The listing builds one solid part. Answer for the finished solid, in the listing's coordinates (mm). Face numbers are marked on the shaded views. Give positions to 0.01 mm unless a question says otherwise; leave off trailing zeros. Answer in a Markdown table with one row per item.
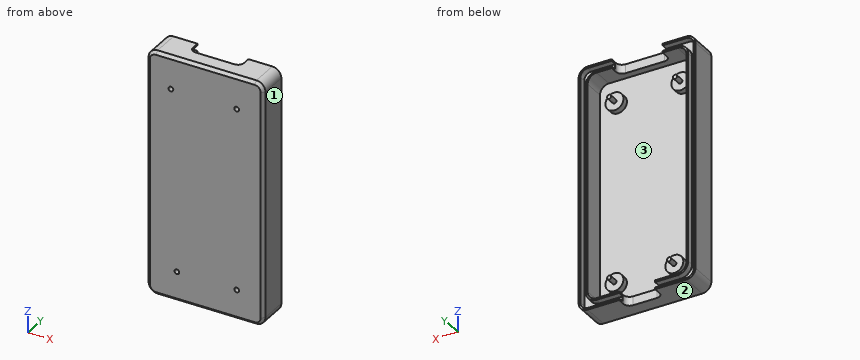
from build123d import *

# Parameters (mm, degrees)
SKETCH1_W                       = 39
SKETCH1_H                       = 81.75
SKETCH1_R                       = 3
BOSS_EXTRUDE1_DEPTH             = 3
SKETCH3_W                       = 39
SKETCH3_H                       = 81.75
SKETCH3_W_2                     = 33
SKETCH3_H_2                     = 75.75
BOSS_EXTRUDE3_DEPTH             = 5
BOSS_EXTRUDE4_START             = 3
SKETCH1_3_R                     = 3
BOSS_EXTRUDE4_DEPTH             = 2
SKETCH8_R                       = 0.7
BOARD_MOUNTING_STANDOFFS_DEPTH  = 3
TAP_DRILL_FOR_M2X0_4_TAP1_D     = 1.6
TAP_DRILL_FOR_M2X0_4_TAP1_DEPTH = 4.519311505
TAP_DRILL_FOR_M2X0_4_TAP1_TIP   = 0.480688495
FILLET2_R                       = 3
SKETCH6_W                       = 12
SKETCH6_H                       = 3
SKETCH6_W_2                     = 17
CUT_EXTRUDE1_DEPTH              = 2.5
STANDOFFS1_LIP_START            = 8
STANDOFFS1_LIP_DEPTH            = 2
STANDOFFS2_LIP_START            = 8
STANDOFFS2_LIP_DEPTH            = 2
FILLET4_R                       = 2
CHAMFER1_SIZE                   = 1


with BuildPart() as part:
    # Sketch1 → Boss-Extrude1 (new body)
    # profile 1 of 5: a face of its own
    with BuildSketch(Plane(origin=(0, 0, 0), x_dir=(1, 0, 0), z_dir=(0, 1, 0))):
        with Locations((14.5, 35.875)):
            Rectangle(SKETCH1_W, SKETCH1_H)
        with Locations((3, 6)):
            Circle(SKETCH1_R, mode=Mode.SUBTRACT)
        with Locations((25, 6)):
            Circle(SKETCH1_R, mode=Mode.SUBTRACT)
        with Locations((5, 66.75)):
            Circle(SKETCH1_R, mode=Mode.SUBTRACT)
        with Locations((25, 66.75)):
            Circle(SKETCH1_R, mode=Mode.SUBTRACT)
    # profile 2 of 5: a face of its own
    with BuildSketch(Plane(origin=(0, 0, 0), x_dir=(1, 0, 0), z_dir=(0, 1, 0))):
        with Locations((5, 66.75)):
            Circle(SKETCH1_R)
    # profile 3 of 5: a face of its own
    with BuildSketch(Plane(origin=(0, 0, 0), x_dir=(1, 0, 0), z_dir=(0, 1, 0))):
        with Locations((25, 66.75)):
            Circle(SKETCH1_R)
    # profile 4 of 5: a face of its own
    with BuildSketch(Plane(origin=(0, 0, 0), x_dir=(1, 0, 0), z_dir=(0, 1, 0))):
        with Locations((25, 6)):
            Circle(SKETCH1_R)
    # profile 5 of 5: a face of its own
    with BuildSketch(Plane(origin=(0, 0, 0), x_dir=(1, 0, 0), z_dir=(0, 1, 0))):
        with Locations((3, 6)):
            Circle(SKETCH1_R)
    extrude(amount=BOSS_EXTRUDE1_DEPTH)

    # Sketch3 → Boss-Extrude3 (add)
    with BuildSketch(Plane(origin=(0, 3, 0), x_dir=(1, 0, 0), z_dir=(0, 1, 0))):
        with Locations((14.5, 35.875)):
            Rectangle(SKETCH3_W, SKETCH3_H)
        with Locations((14.5, 35.875)):
            Rectangle(SKETCH3_W_2, SKETCH3_H_2, mode=Mode.SUBTRACT)
    extrude(amount=BOSS_EXTRUDE3_DEPTH)

    # Sketch1<3> → Boss-Extrude4 (add)
    with BuildSketch(Plane(origin=(0, 0, 0), x_dir=(1, 0, 0), z_dir=(0, 1, 0)).offset(BOSS_EXTRUDE4_START)):
        with Locations(Location((3, 6, 0), (0, 0, 270))):
            Circle(SKETCH1_3_R)
        with Locations(Location((25, 6, 0), (0, 0, 270))):
            Circle(SKETCH1_3_R)
        with Locations(Location((25, 66.75, 0), (0, 0, 270))):
            Circle(SKETCH1_3_R)
        with Locations(Location((5, 66.75, 0), (0, 0, 270))):
            Circle(SKETCH1_3_R)
    extrude(amount=BOSS_EXTRUDE4_DEPTH)

    # Sketch8 → Board Mounting Standoffs (add)
    with BuildSketch(Plane(origin=(0, 5, 0), x_dir=(1, 0, 0), z_dir=(0, 1, 0))):
        with Locations(Location((5, 66.75, 0), (0, 0, 270))):
            Circle(SKETCH8_R)
        with Locations(Location((25, 66.75, 0), (0, 0, 270))):
            Circle(SKETCH8_R)
        with Locations(Location((3, 6, 0), (0, 0, 270))):
            Circle(SKETCH8_R)
        with Locations(Location((25, 6, 0), (0, 0, 270))):
            Circle(SKETCH8_R)
    extrude(amount=BOARD_MOUNTING_STANDOFFS_DEPTH)

    # Tap Drill for M2x0.4 Tap1
    with Locations(Plane(origin=(0, 0, 0), x_dir=(-1, 0, 0), z_dir=(0, -1, 0))):
        with Locations((-25, 66.75), (-5, 66.75), (-25, 6), (-3, 6)):
            Hole(TAP_DRILL_FOR_M2X0_4_TAP1_D / 2, depth=TAP_DRILL_FOR_M2X0_4_TAP1_DEPTH)
            with Locations((0, 0, -(TAP_DRILL_FOR_M2X0_4_TAP1_DEPTH + TAP_DRILL_FOR_M2X0_4_TAP1_TIP / 2))):  # 118° drill point
                Cone(0, TAP_DRILL_FOR_M2X0_4_TAP1_D / 2, TAP_DRILL_FOR_M2X0_4_TAP1_TIP, mode=Mode.SUBTRACT)

    # Fillet2
    fillet2_edges = [part.edges().sort_by_distance(p)[0] for p in [
        (-2, 5.5, -73.75),
        (-2, 5.5, 2),
        (31, 5.5, 2),
        (31, 5.5, -73.75),
        (-5, 4, -76.75),
        (34, 4, -76.75),
        (34, 4, 5),
        (-5, 4, 5),
    ]]
    fillet(fillet2_edges, radius=FILLET2_R)

    # Sketch6 → Cut-Extrude1 (cut)
    with BuildSketch(Plane(origin=(0, 8, 0), x_dir=(1, 0, 0), z_dir=(0, 1, 0))):
        with Locations((14.5, 75.25)):
            Rectangle(SKETCH6_W, SKETCH6_H)
        with Locations((14.5, -3.5)):
            Rectangle(SKETCH6_W_2, SKETCH6_H)
    extrude(amount=-CUT_EXTRUDE1_DEPTH, mode=Mode.SUBTRACT)

    # Standoffs1-Lip: read off the stored shape, not the designer's step
    # Standoffs1-Lip outline → Standoffs1-Lip (add)
    with BuildSketch(Plane(origin=(0, 0, 0), x_dir=(1, 0, 0), z_dir=(0, 1, 0)).offset(STANDOFFS1_LIP_START)):
        with BuildLine():
            Line((23, -5), (31, -5))
            ThreePointArc((31, -5), (33.121320344, -4.121320344), (34, -2))
            Line((34, -2), (34, 73.75))
            ThreePointArc((34, 73.75), (33.121320344, 75.871320344), (31, 76.75))
            Line((31, 76.75), (20.5, 76.75))
            Line((20.5, 76.75), (20.5, 73.75))
            Line((20.5, 73.75), (28, 73.75))
            ThreePointArc((28, 73.75), (30.121320344, 72.871320344), (31, 70.75))
            Line((31, 70.75), (31, 1))
            ThreePointArc((31, 1), (30.121320344, -1.121320344), (28, -2))
            Line((28, -2), (23, -2))
            Line((23, -2), (23, -5))
        make_face()
    extrude(amount=STANDOFFS1_LIP_DEPTH)

    # Standoffs1-Lip 2: loft between two sections, ruled curve by curve
    standoffs1_lip_2_from = [
        Edge.make_three_point_arc((33.3, 8, -73.75), (32.626345597, 8, -75.376345597), (31, 8, -76.05)),
        Edge.make_three_point_arc((31, 8, 4.3), (32.626345597, 8, 3.626345597), (33.3, 8, 2)),
        Edge.make_three_point_arc((31.7, 8, -1), (30.61629509, 8, 1.61629509), (28, 8, 2.7)),
        Edge.make_three_point_arc((28, 8, -74.45), (30.61629509, 8, -73.36629509), (31.7, 8, -70.75)),
        Edge.make_line((20.5, 8, -76.05), (31, 8, -76.05)),
        Edge.make_line((33.3, 8, -73.75), (33.3, 8, 2)),
        Edge.make_line((31, 8, 4.3), (23, 8, 4.3)),
        Edge.make_line((20.5, 8, -74.45), (28, 8, -74.45)),
        Edge.make_line((28, 8, 2.7), (23, 8, 2.7)),
        Edge.make_line((31.7, 8, -70.75), (31.7, 8, -1)),
        Edge.make_line((20.5, 8, -74.45), (20.5, 8, -76.05)),
        Edge.make_line((23, 8, 2.7), (23, 8, 4.3)),
    ]
    standoffs1_lip_2_to = [
        Edge.make_three_point_arc((33.404815559, 10, -73.75), (32.700461389, 10, -75.450461389), (31, 10, -76.154815559)),
        Edge.make_three_point_arc((31, 10, 4.404815559), (32.700461389, 10, 3.700461389), (33.404815559, 10, 2)),
        Edge.make_three_point_arc((31.595184441, 10, -1), (30.542179298, 10, 1.542179298), (28, 10, 2.595184441)),
        Edge.make_three_point_arc((28, 10, -74.345184441), (30.542179298, 10, -73.292179298), (31.595184441, 10, -70.75)),
        Edge.make_line((20.5, 10, -76.154815559), (31, 10, -76.154815559)),
        Edge.make_line((33.404815559, 10, -73.75), (33.404815559, 10, 2)),
        Edge.make_line((31, 10, 4.404815559), (23, 10, 4.404815559)),
        Edge.make_line((20.5, 10, -74.345184441), (28, 10, -74.345184441)),
        Edge.make_line((28, 10, 2.595184441), (23, 10, 2.595184441)),
        Edge.make_line((31.595184441, 10, -70.75), (31.595184441, 10, -1)),
        Edge.make_line((20.5, 10, -74.345184441), (20.5, 10, -76.154815559)),
        Edge.make_line((23, 10, 2.595184441), (23, 10, 4.404815559)),
    ]
    standoffs1_lip_2 = Solid(Shell([*[Face.make_surface_from_curves(standoffs1_lip_2_from[k], standoffs1_lip_2_to[k]) for k in range(12)], Face(Wire(standoffs1_lip_2_from)), Face(Wire(standoffs1_lip_2_to))]))
    add(standoffs1_lip_2, mode=Mode.SUBTRACT)

    # Standoffs2-Lip: read off the stored shape, not the designer's step
    # Standoffs2-Lip outline → Standoffs2-Lip (add)
    with BuildSketch(Plane(origin=(0, 0, 0), x_dir=(1, 0, 0), z_dir=(0, 1, 0)).offset(STANDOFFS2_LIP_START)):
        with BuildLine():
            ThreePointArc((-2, 76.75), (-4.121320344, 75.871320344), (-5, 73.75))
            Line((-5, 73.75), (-5, -2))
            ThreePointArc((-5, -2), (-4.121320344, -4.121320344), (-2, -5))
            Line((-2, -5), (6, -5))
            Line((6, -5), (6, -2))
            Line((6, -2), (1, -2))
            ThreePointArc((1, -2), (-1.121320344, -1.121320344), (-2, 1))
            Line((-2, 1), (-2, 70.75))
            ThreePointArc((-2, 70.75), (-1.121320344, 72.871320344), (1, 73.75))
            Line((1, 73.75), (8.5, 73.75))
            Line((8.5, 73.75), (8.5, 76.75))
            Line((8.5, 76.75), (-2, 76.75))
        make_face()
    extrude(amount=STANDOFFS2_LIP_DEPTH)

    # Standoffs2-Lip 2: loft between two sections, ruled curve by curve
    standoffs2_lip_2_from = [
        Edge.make_three_point_arc((-4.3, 8, 2), (-3.626345597, 8, 3.626345597), (-2, 8, 4.3)),
        Edge.make_three_point_arc((-2, 8, -76.05), (-3.626345597, 8, -75.376345597), (-4.3, 8, -73.75)),
        Edge.make_three_point_arc((-2.7, 8, -70.75), (-1.61629509, 8, -73.36629509), (1, 8, -74.45)),
        Edge.make_three_point_arc((1, 8, 2.7), (-1.61629509, 8, 1.61629509), (-2.7, 8, -1)),
        Edge.make_line((-2, 8, -76.05), (8.5, 8, -76.05)),
        Edge.make_line((6, 8, 4.3), (-2, 8, 4.3)),
        Edge.make_line((1, 8, -74.45), (8.5, 8, -74.45)),
        Edge.make_line((6, 8, 2.7), (1, 8, 2.7)),
        Edge.make_line((-4.3, 8, 2), (-4.3, 8, -73.75)),
        Edge.make_line((-2.7, 8, -1), (-2.7, 8, -70.75)),
        Edge.make_line((8.5, 8, -74.45), (8.5, 8, -76.05)),
        Edge.make_line((6, 8, 2.7), (6, 8, 4.3)),
    ]
    standoffs2_lip_2_to = [
        Edge.make_three_point_arc((-4.404815559, 10, 2), (-3.700461389, 10, 3.700461389), (-2, 10, 4.404815559)),
        Edge.make_three_point_arc((-2, 10, -76.154815559), (-3.700461389, 10, -75.450461389), (-4.404815559, 10, -73.75)),
        Edge.make_three_point_arc((-2.595184441, 10, -70.75), (-1.542179298, 10, -73.292179298), (1, 10, -74.345184441)),
        Edge.make_three_point_arc((1, 10, 2.595184441), (-1.542179298, 10, 1.542179298), (-2.595184441, 10, -1)),
        Edge.make_line((-2, 10, -76.154815559), (8.5, 10, -76.154815559)),
        Edge.make_line((6, 10, 4.404815559), (-2, 10, 4.404815559)),
        Edge.make_line((1, 10, -74.345184441), (8.5, 10, -74.345184441)),
        Edge.make_line((6, 10, 2.595184441), (1, 10, 2.595184441)),
        Edge.make_line((-4.404815559, 10, 2), (-4.404815559, 10, -73.75)),
        Edge.make_line((-2.595184441, 10, -1), (-2.595184441, 10, -70.75)),
        Edge.make_line((8.5, 10, -74.345184441), (8.5, 10, -76.154815559)),
        Edge.make_line((6, 10, 2.595184441), (6, 10, 4.404815559)),
    ]
    standoffs2_lip_2 = Solid(Shell([*[Face.make_surface_from_curves(standoffs2_lip_2_from[k], standoffs2_lip_2_to[k]) for k in range(12)], Face(Wire(standoffs2_lip_2_from)), Face(Wire(standoffs2_lip_2_to))]))
    add(standoffs2_lip_2, mode=Mode.SUBTRACT)

    # Fillet4
    fillet4_edges = [part.edges().sort_by_distance(p)[0] for p in [
        (8.5, 5.5, -75.25),
        (20.5, 5.5, -75.25),
        (6, 5.5, 3.5),
        (23, 5.5, 3.5),
    ]]
    fillet(fillet4_edges, radius=FILLET4_R)

    # Chamfer1
    chamfer1_edges = [part.edges().sort_by_distance(p)[0] for p in [
        (34, 0, -35.875),
        (-5, 0, -35.875),
        (14.5, 0, -76.75),
        (14.5, 0, 5),
        (33.121320344, 0, -75.871320344),
        (-4.121320344, 0, -75.871320344),
        (-4.121320344, 0, 4.121320344),
        (33.121320344, 0, 4.121320344),
    ]]
    chamfer(chamfer1_edges, length=CHAMFER1_SIZE)


solid = part.part
Item 1: Each of these flat-tipped pins is pushed along its axis until it touches: P1, Ø5, axis at x = 24.5, z = -68, coming from the +Y side; P2, Ø2.5, axis at x = 16, z = -75.5, coming from the +Y side; P3, Ø4, axis at x = 17.5, z = -25, coming from the +Y side. Where does it stop, or does it pass through?
Answer block:
| item | result |
|---|---|
| P1 | y = 8 |
| P2 | y = 5.5 |
| P3 | y = 3 |
Item 2: Consider line 1 (Z direction, x = 25, y = 1.75); line 2 (X direction, y = 9.75, z = -56); line 3 (X direction, y = 2.5, z = -6). Determine where each line is inside the solid, lowest interval first.
Answer block:
| item | result |
|---|---|
| line 1 | -76.75 to -67.55, -65.95 to -6.8, -5.2 to 5 |
| line 2 | -5 to -4.39, -2.61 to -2, 31 to 31.61, 33.39 to 34 |
| line 3 | -5 to 2.2, 3.8 to 24.2, 25.8 to 34 |
Item 3: Determine the mould class of the marked faces 1, 2 and 3 for opening direction Z: pulls with the +Z half, pulls with the -Z half, needs draft (parallel to the pull), parting line crosses it, or undercut.
Answer block:
| item | result |
|---|---|
| face 1 | needs draft |
| face 2 | pulls with the -Z half |
| face 3 | undercut |
